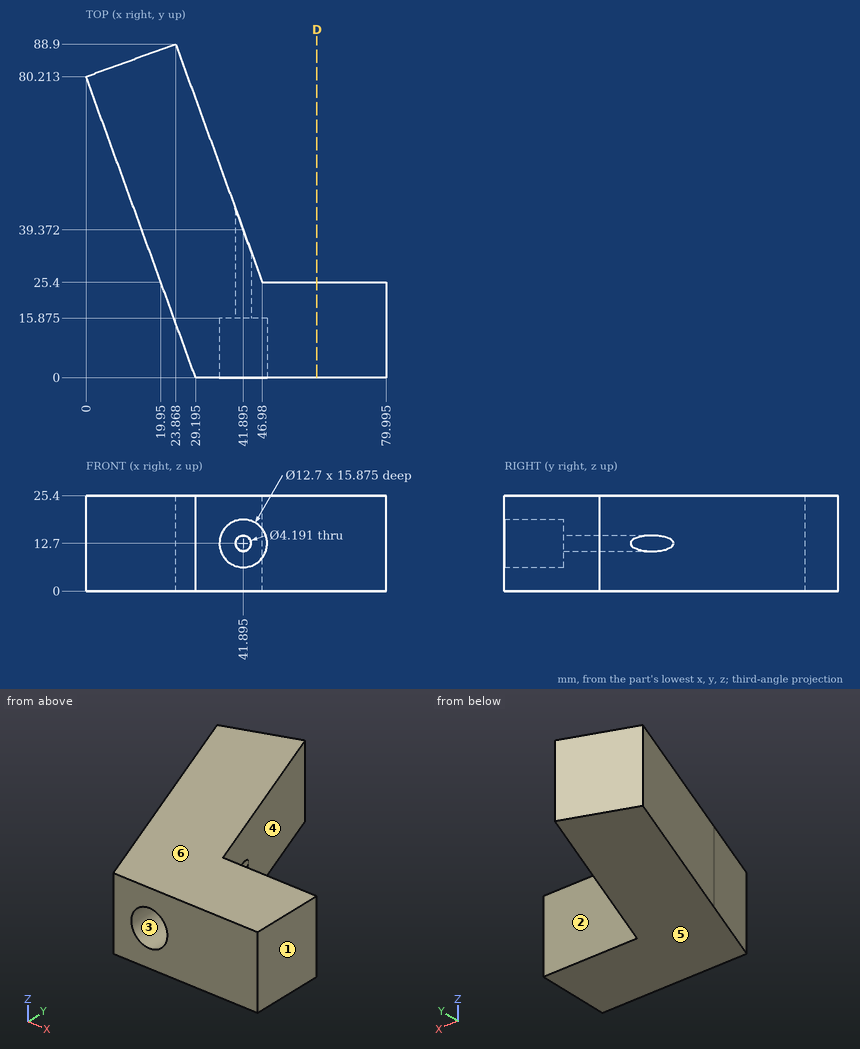
Design review of the part shown in the three views and the two pictorial views. Dimensions are in mm from the part's minimum x, y and z. A direction names the side the tool comes from. Round coordinates to 2 decimals unless told otherwise and drop trailing zeros. Order: outer loops, then holes, each group sorted by start corner. A loop starts at its lowest first (then second) coordinate and runs counter-clockwise, first axis right, second up. Notation, with made-up numbers: M -32.75,27.25 L -6.75,27.25 A26 cw -6.75,42.25 Z; hole C -9,46.25 d3. An arc over 180 degrees is marked long. Put each result on its own line as item: value.
Q1. Consider section D-D (x = 61.5). State the section outline as (y, z) points, and give its area (3 significant figures).
Reported:
outline: M 0,0 L 25.4,0 L 25.4,25.4 L 0,25.4 Z
area: 645 mm²
Q2. To check wall thickness, follow line 1 (X direction, y = 4.5, z = 12.7) (1 decimal); line 2 (Y direction, x = 50, z = 19); line 3 (X direction, y = 9, z = 12.7) (1 decimal). State the ranges of each line that lie inside material, in increasing order.
Reported:
line 1: 27.6 to 35.5, 48.2 to 80
line 2: 0 to 25.4
line 3: 25.9 to 35.5, 48.2 to 80
Q3. Machinability: for the marked faces 1 and 2, which of the approach directions +Z, -Z, +X, -X, +Y, -Y give a long, thin tool a straight path to every point of the face, cutting with its end or side? Answer none if there is none.
Reported:
face 1: +Z, -Z, +X, +Y, -Y
face 2: +Z, -Z, +X, +Y
Q4. Insertion check: pin 1 Ø4 at (x, z) = (41.9, 12.7) entering from +Y; pin 2 Ø1 at (x, z) = (67, 3.5) entering from +Y; pin 3 Ø6.5 at (x, z) = (42, 12) entering from -Y (3 decimals); pin 4 Ø10 at (y, z) = (68.5, 6) entering from -X. Each pin has a flat end and moves straight along its axis. Give the tip position at first contact, or say it passes through.
Reported:
pin 1: through
pin 2: y = 25.4
pin 3: y = 15.875
pin 4: x = 2.44
Q5. Draft analysis for pull direction Z (two halves, no side actions). For the marked faces 3, 4, 5 and 6, state which applies: released by +Z, released by -Z, zero draft, split by the parting line, or undercut.
Reported:
face 3: undercut
face 4: zero draft
face 5: released by -Z
face 6: released by +Z
